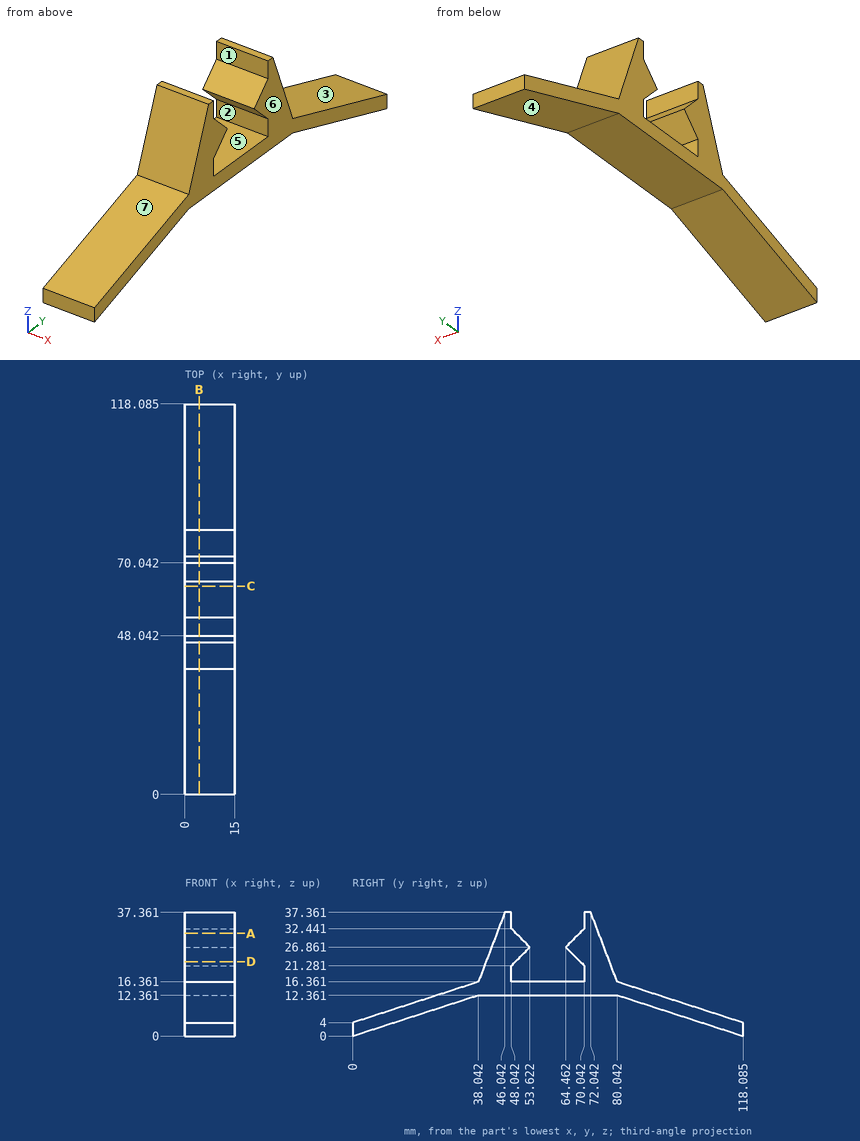
The drawing under review shows one solid part. Ordinate dimensions are in mm from its lowest x, y, z. A direction names the side the tool comes from. Round coordinates to 2 decimals unless told otherwise and drop trailing zeros. Loops run counter-clockwise (first coordinate to the right, second up) from the corner with the lowest first, then second, coordinate; pieces in that order, holes last. Notation, with made-up numbers: M -29,-36 L 14,-36 A37 cw 14,2 Z; hole C 85.5,77 d5. An arc over 180 degrees is marked long. Answer as CSV lines item,"result". Start each with the question number.
Item 1: For the marked faces 1, 2, 3 and 4, list the 3-axis set-ups (+Z, -Z, +X, -X, +Y, -Y) from which the entire face can be reached by the end or side of a thin tool; tool diameter is ignored.
Item 2: Consider section C-C (y = 63). Write out the cut boundary in (x, z).
Item 3: Insertion check: P1, Ø5, axis at x = 3, y = 41.5, coming from the -Z side; P2, Ø5, axis at y = 50, z = 16, coming from the -X side; P3, Ø2.5, axis at x = 7, z = 36, coming from the -Y side; P4, Ø2.5, axis at x = 8, z = 19.5, coming from the +Y side. Each pin has a flat end and moves straight along its axis. Give the tip position at first contact, or say it passes through.
Item 4: Mouldability with a two-part tool opening along Y and no side actions: class the marked faces 5, 6 and 7 as released by +Y, released by -Y, zero draft, split by the parting line, or undercut.
Item 5: Consider section B-B (x = 4.25). Write out the cut boundary in (y, z) (1 decimal).
Item 6: Wall thickness on line 1 (Y direction, x = 3.5, z = 23.5) (1 decimal); line 2 (Y direction, x = 2.25, z = 29) (1 decimal); line 3 (Z direction, x = 8, y = 68.5) (1 decimal): over which ranges is each line inside the solid? List them lowest first. Write a range as [from, to].
Item 7: Consider section A-A (z = 31). Write out the cut boundary in (x, y) (1 decimal), then the cut area to 3 significant figures.
Item 8: Consider section D-D (z = 22.5). Write out the cut boundary in (x, y).
Answer:
1,face 1,"+Z, +X, -X"
1,face 2,"+X, -X"
1,face 3,"+Z, +X, -X, +Y"
1,face 4,"-Z, +X, -X"
2,outline,"M 0,12.36 L 15,12.36 L 15,16.36 L 0,16.36 Z"
3,P1,"stops at z = 12.36"
3,P2,"stops at x = 0"
3,P3,"stops at y = 45.05"
3,P4,"stops at y = 79.32"
4,face 5,"undercut"
4,face 6,"zero draft"
4,face 7,"released by -Y"
5,outline,"M 0,0 L 38,12.4 L 80,12.4 L 118.1,0 L 118.1,4 L 80,16.4 L 72,37.4 L 70,37.4 L 70,32.4 L 64.5,26.9 L 70,21.3 L 70,16.4 L 48,16.4 L 48,21.3 L 53.6,26.9 L 48,32.4 L 48,37.4 L 46,37.4 L 38,16.4 L 0,4 Z"
6,line 1,"y = [40.8, 50.3], [67.8, 77.3]"
6,line 2,"y = [42.9, 51.5], [66.6, 75.2]"
6,line 3,"z = [12.4, 16.4], [22.8, 30.9]"
7,outline,"M 0,43.6 L 15,43.6 L 15,49.5 L 0,49.5 Z; M 0,68.6 L 15,68.6 L 15,74.5 L 0,74.5 Z"
7,area,"176 mm^2"
8,outline,"M 0,40.38 L 15,40.38 L 15,49.26 L 0,49.26 Z; M 0,68.82 L 15,68.82 L 15,77.7 L 0,77.7 Z"
